Work out the finished part from the listing and answer in its coordinate system (mm). A direction names the side the tool comes from. Coordinates: 2 decimals unless noted, no trailing zeros. Order: outer loops, then holes, each group sorted by start corner. A loop starts at its lowest first (then second) coordinate and runs counter-clockwise, first axis right, second up. Notation, with made-up numbers: M -31,42.5 L 5,42.5 A30 cw 5,70.5 Z; hole C -17.75,48 d5. An arc over 180 degrees is marked long. Use a Markdown table: item, result.
from build123d import *

# Parameters (mm, degrees)
SKETCH_1_W          = 80
SKETCH_1_H          = 55
EXTRUDE_1_DEPTH     = 3
SKETCH_2_R          = 1.55
CUT_EXTRUDE_1_DEPTH = 24.5
SKETCH_3_W          = 3
SKETCH_3_H          = 55
EXTRUDE_2_DEPTH     = 1.5
SKETCH_5_W          = 3
SKETCH_5_H          = 55
EXTRUDE_3_DEPTH     = 50
SKETCH_6_W          = 51.5
SKETCH_6_H          = 3
EXTRUDE_4_DEPTH     = 50
SKETCH_7_W          = 51.5
SKETCH_7_H          = 3
EXTRUDE_5_DEPTH     = 50
SKETCH_8_W          = 51.5
SKETCH_8_H          = 155
EXTRUDE_6_DEPTH     = 40
EXTRUDE_7_DEPTH     = 12
CUT_EXTRUDE_2_DEPTH = 184
SKETCH_13_R         = 90
CUT_EXTRUDE_3_DEPTH = 92
SKETCH_14_W         = 68
SKETCH_14_H         = 37
EXTRUDE_8_DEPTH     = 40


with BuildPart() as part:
    # Sketch 1 → Extrude 1 (new body)
    with BuildSketch(Plane.XY):
        Rectangle(SKETCH_1_W, SKETCH_1_H)
    extrude(amount=EXTRUDE_1_DEPTH)

    # Sketch 2 → Cut-Extrude 1 (cut)
    with BuildSketch(Plane(origin=(0, 0, 0), x_dir=(-1, 0, 0), z_dir=(0, 0, -1))):
        with Locations((37, 25)):
            Circle(SKETCH_2_R)
        with Locations((37, -25)):
            Circle(SKETCH_2_R)
        with Locations((-13, 25)):
            Circle(SKETCH_2_R)
        with Locations((-13, -25)):
            Circle(SKETCH_2_R)
    extrude(amount=-CUT_EXTRUDE_1_DEPTH, mode=Mode.SUBTRACT)



with BuildPart() as body_2:
    # Sketch 3 → Extrude 2 (new body)
    with BuildSketch(Plane(origin=(40, 0, 0), x_dir=(0, 0, -1), z_dir=(1, 0, 0))):
        with Locations((-1.5, 0)):
            Rectangle(SKETCH_3_W, SKETCH_3_H)
    extrude(amount=EXTRUDE_2_DEPTH)

    # Sketch 5 → Extrude 3 (add)
    with BuildSketch(Plane(origin=(41.5, 0, 0), x_dir=(0, 0, -1), z_dir=(1, 0, 0))):
        with Locations((-1.5, 0)):
            Rectangle(SKETCH_5_W, SKETCH_5_H)
    extrude(amount=EXTRUDE_3_DEPTH)


with BuildPart() as part_1:
    add(part.part)

    add(body_2.part)  # Extrude 4 merges body 2
    # Sketch 6 → Extrude 4 (add)
    with BuildSketch(Plane(origin=(0, 27.5, 0), x_dir=(1, 0, 0), z_dir=(0, 1, 0))):
        with Locations((65.75, -1.5)):
            Rectangle(SKETCH_6_W, SKETCH_6_H)
    extrude(amount=EXTRUDE_4_DEPTH)

    # Sketch 7 → Extrude 5 (add)
    with BuildSketch(Plane.XZ.offset(27.5)):
        with Locations((65.75, 1.5)):
            Rectangle(SKETCH_7_W, SKETCH_7_H)
    extrude(amount=EXTRUDE_5_DEPTH)

    # Sketch 8 → Extrude 6 (add)
    with BuildSketch(Plane(origin=(0, 0, 0), x_dir=(-1, 0, 0), z_dir=(0, 0, -1))):
        with Locations((-65.75, 0)):
            Rectangle(SKETCH_8_W, SKETCH_8_H)
    extrude(amount=EXTRUDE_6_DEPTH)

    # Sketch 9 → Extrude 7 (add)
    with BuildSketch(Plane.ZY.offset(-40)):
        Polygon((-40, 39.5), (3, 39.5), (3, 27.5), (0, 27.5), (0, -27.5), (3, -27.5), (3, -39.5), (-40, -39.5), align=None)
    extrude(amount=EXTRUDE_7_DEPTH)

    # Sketch 10 → Cut-Extrude 2 (cut)
    with BuildSketch(Plane(origin=(0, 77.5, 0), x_dir=(1, 0, 0), z_dir=(0, 1, 0))):
        Polygon((56.5, 12), (91.5, -3), (50.071428571, -3), align=None)
    extrude(amount=-CUT_EXTRUDE_2_DEPTH, mode=Mode.SUBTRACT)

    # Sketch 13 → Cut-Extrude 3 (cut, symmetric)
    with BuildSketch(Plane(origin=(13.112068966, 0, -30.594827586), x_dir=(0.9191450300180579, 0, 0.39391929857916774), z_dir=(-0.39391929857916774, 0, 0.9191450300180579))):
        with Locations((120.283528142, 0)):
            Circle(SKETCH_13_R)
    extrude(amount=CUT_EXTRUDE_3_DEPTH, both=True, mode=Mode.SUBTRACT)

    # Sketch 14 → Extrude 8 (add)
    with BuildSketch(Plane(origin=(0, 0, 0), x_dir=(-1, 0, 0), z_dir=(0, 0, -1))):
        with Locations((6, 0)):
            Rectangle(SKETCH_14_W, SKETCH_14_H)
    extrude(amount=EXTRUDE_8_DEPTH)


solid = part_1.part
(1) A cutting plane is placed at B-B (y = 66). Determine the outline of the cut face in (x, z).
Conclusion:
| item | result |
|---|---|
| outline | M 40,-40 L 81.44,-40 L 67.43,-7.32 L 56.5,-12 L 50.07,3 L 40,3 Z |
(2) Which of the six approach directions +Z, -Z, +X, -X, +Y, -Y give full straight-line access (tool end or side, diameter ignored) to faces 4 (the flat face through (-6, 23, 0)), 5 (the flat face through (40, -59, -18)), 6 (the flat face through (63.3, -70.389, -9.086))?
Conclusion:
| item | result |
|---|---|
| face 4 | -Z, -X, +Y |
| face 5 | +Z, -Z, -X, -Y |
| face 6 | +Z, +Y, -Y |
(3) Straight lines are drawn through the part: L1, parallel to Y at x = 13, z = 1; L2, parallel to Y at x = 5.5, z = -36; L3, parallel to Y at x = 61, z = -34.5. For each, find the intervals that lie inside material, in ascending order.
Conclusion:
| item | result |
|---|---|
| L1 | -27.5 to -26.55, -23.45 to 23.45, 26.55 to 27.5 |
| L2 | -18.5 to 18.5 |
| L3 | -77.5 to -45.24, 45.24 to 77.5 |
(4) A cutting plane is placed at A-A (x = -2). Determine the outline of the cut face in (y, z), then the cut area to 4 significant figures.
Conclusion:
| item | result |
|---|---|
| outline | M -27.5,0 L -18.5,0 L -18.5,-40 L 18.5,-40 L 18.5,0 L 27.5,0 L 27.5,3 L -27.5,3 Z |
| area | 1,645 mm2 |
(5) Determine the mould class of faces 1 (the flat face through (5, 0, 3)), 2 (the flat face through (-40, 0, -19)), 3 (the flat face through (63.3, 70.739, -9.086)) for opening direction X: pulls with the +X half, pulls with the -X half, needs draft (parallel to the pull), parting line crosses it, or undercut.
Conclusion:
| item | result |
|---|---|
| face 1 | needs draft |
| face 2 | pulls with the -X half |
| face 3 | undercut |
(6) A cutting plane is placed at C-C (y = -50.5). Determine the outline of the cut face in (x, z), then the cut area to 3 significant figures.
Conclusion:
| item | result |
|---|---|
| outline | M 40,-40 L 66.96,-40 L 48.53,3 L 40,3 Z |
| area | 763 mm2 |
(7) Given P1, Ø1.9, axis at x = -37, y = -25, coming from the -Z side; P2, Ø13, axis at x = 34.5, z = -21, coming from the -Y side; P3, Ø4, axis at x = 17, z = -32.5, coming from the +Y side; P4, Ø6.5, axis at y = 28, z = -24, coming from the -X side, each flat-ended and moving along its own axis, determine where each tip first touches the part or whether it passes through.
Conclusion:
| item | result |
|---|---|
| P1 | through |
| P2 | y = -77.5 |
| P3 | y = 18.5 |
| P4 | x = 28 |
